Part model, mm, in its own coordinate system. A direction names the side the tool comes from. Coordinates: 2 decimals unless noted, no trailing zeros. Loops run counter-clockwise (first coordinate to the right, second up) from the corner with the lowest first, then second, coordinate; pieces in that order, holes last. Notation, with made-up numbers: (77.5, 22) - (98.5, 22) arc R32 ccw to (98.5, 48) - close; hole circle Ø9 at (81.5, -14.5). An arc over 180 degrees is marked (long way). Use a Markdown table: item, result. Add a question column.
1) Probe probe 1 along Z at (x, y) = (3, -5.5); probe 2 along Z at (x, y) = (-9, 2.75); probe 3 along Y at (x, z) = (-7, 4.5). List the from-to ranges inside material, lowest first. Write a range as [from, to].
2) Band-saw the part on B-B (z = -0.5). Give the cut face in (x, y).
3) Band-saw the part on C-C (x = -8). Give the cut face in (y, z).
4) Band-saw the part on A-A (z = -6.5). Give the cut face in (x, y), plus the area to 3 significant figures.
5) Drop flat-ended pins along their axis: P1, Ø1.1, axis at y = -2.5, z = 7.5, coming from the -X side; P2, Ø1, axis at x = -2, z = -0.5, coming from the -Y side; P3, Ø2.5, axis at x = -8, z = 5.5, coming from the +Y side. Give the stop position or say it passes through.
6) Pull direction X, two halves, no side cores. Call faces 1 (the face through (-11.75, -4, 0)), 2 (the face through (7, -4, 4)), 3 (the face through (-4, 1, -3)): +X half, -X half, draft (parallel to the pull), parting line (faces both ways), or undercut.
7) Tool access for faces 4 (the face through (-3.94, 1.79, -5.46)), 5 (the face through (6.036, -4.5, 7.5)), 6 (the face through (0.75, 4, -6)), 7 (the face through (1.65, 7.39, -5.46)): list every direction of +Z, -Z, +X, -X, +Y, -Y with a clear straight run to the whole face (end or side of a thin tool).
Autodesk Inventor part; units mm, degrees
ref_plane "YZ Plane" through (0, 0, 0) normal (1, 0, 0) x (0, 1, 0)
ref_plane "XZ Plane" through (0, 0, 0) normal (0, 1, 0) x (-1, 0, 0)
ref_plane "XY Plane" through (0, 0, 0) normal (0, 0, 1) x (1, 0, 0)
sketch "스케치1" plane through (0, 0, 0) normal (0, 0, 1) x (1, 0, 0)
  line L0 (-11.75, 8.25) -> (11.75, 8.25)
  line L1 (11.75, 8.25) -> (11.75, -8.25)
  line L2 (11.75, -8.25) -> (-11.75, -8.25)
  line L3 (-11.75, -8.25) -> (-11.75, 8.25)
  line L4 (-11.75, 8.25) -> (11.75, -8.25) construction
  line L5 (11.75, 8.25) -> (-11.75, -8.25) construction
  line L6 (-11.75, -4.25) -> (0.75, -4.25)
  line L7 (0.75, -4.25) -> (0.75, 8.25)
  circle A0 centre (-6.25, 2.75) radius 2.5
  point P0 (0, 0)
  dimension "d0" = 23.5
  dimension "d1" = 16.5
  dimension "d3" = 4
  dimension "d4" = 12.5
  dimension "d5" = 5
  dimension "d6" = 11
  dimension "d7" = 18
extrude "돌출1" add sketch "스케치1" along normal mid plane 16 contours L0 L1 L2 L3 L6 L7 | A0
extrude "돌출2" add sketch "스케치1" along normal mid plane 6 contours L0 L7 L6 L3
ref_plane "작업 평면1" through (0, 0, 0) normal (0, 0, 1) x (1, 0, 0)
sketch "스케치2" plane through (0, 0, 0) normal (0, 0, 1) x (1, 0, 0)
  line L0 (11.75, 8.25) -> (11.75, -8.25)
  line L1 (11.75, 5.75) -> (-3.25, -8.25)
  line L2 (-11.75, -8.25) -> (-11.75, -4.25)
  line L3 (11.75, -8.25) -> (-11.75, -8.25)
  point P0 (0, 0)
  dimension "d12" = 2.5
  dimension "d13" = 8.5
  dimension "d14" = 0
extrude "돌출3" cut sketch "스케치2" along normal mid plane 8
fillet "모깎기1" radius 3 2 edges at (0.75, 8.25, 5.5) (0.75, 8.25, -5.5)
fillet "모깎기2" radius 5.5 1 edges at (-11.75, 8.25, 0)
fillet "모깎기3" radius 7 2 edges at (0.75, -4.25, 5.5) (0.75, -4.25, -5.5)
sketch "스케치3" plane through (0, 0, 8) normal (0, 0, 1) x (1, 0, 0)
  line L0 (0.5954, -0.2053) -> (15.6035, -0.2053) construction
  line L1 (15.6035, -0.2053) -> (15.6035, -10.6024) construction
  line L2 (15.6035, -10.6024) -> (0.5954, -10.6024) construction
  line L3 (0.5954, -10.6024) -> (0.5954, -0.2053) construction
  spline S0 degree 2 poles (0.9131, -2.6219) (0.9131, -2.083) (1.2648, -1.1867) (1.5711, -0.8633) knots 0 0 0 1 2 2 2
  spline S1 degree 2 poles (1.5711, -0.8633) (1.8604, -0.5513) (2.7056, -0.2053) (3.1368, -0.2053) knots 0 0 0 1 2 2 2
  spline S2 degree 2 poles (3.1368, -0.2053) (3.6189, -0.2053) (4.4017, -0.5287) (4.691, -0.835) knots 0 0 0 1 2 2 2
  spline S3 degree 2 poles (4.691, -0.835) (5.0541, -1.2207) (5.4512, -2.4687) (5.4512, -3.4274) knots 0 0 0 1 2 2 2
  spline S4 degree 2 poles (5.4512, -3.4274) (5.4512, -4.2953) (5.0598, -5.8496) (4.6797, -6.3658) knots 0 0 0 1 2 2 2
  spline S5 degree 2 poles (4.6797, -6.3658) (4.2769, -6.9103) (3.1424, -7.4833) (2.3142, -7.4833) knots 0 0 0 1 2 2 2
  spline S6 degree 2 poles (2.3142, -7.4833) (2.127, -7.4833) (1.7016, -7.4436) (1.5201, -7.3868) knots 0 0 0 1 2 2 2
  line L4 (1.5201, -7.3868) -> (1.5201, -6.4849)
  line L5 (1.5201, -6.4849) -> (1.5654, -6.4849)
  spline S7 degree 2 poles (1.5654, -6.4849) (1.6846, -6.553) (2.1838, -6.6721) (2.439, -6.6721) knots 0 0 0 1 2 2 2
  spline S8 degree 2 poles (2.439, -6.6721) (3.358, -6.6721) (4.4074, -5.4582) (4.4812, -4.335) knots 0 0 0 1 2 2 2
  spline S9 degree 2 poles (4.4812, -4.335) (4.1068, -4.5902) (3.4261, -4.8228) (3.0233, -4.8228) knots 0 0 0 1 2 2 2
  spline S10 degree 2 poles (3.0233, -4.8228) (2.6376, -4.8228) (1.9966, -4.6526) (1.6732, -4.4087) knots 0 0 0 1 2 2 2
  spline S11 degree 2 poles (1.6732, -4.4087) (1.2988, -4.1194) (0.9131, -3.2402) (0.9131, -2.6219) knots 0 0 0 1 2 2 2
  spline S12 degree 2 poles (4.5039, -3.2175) (4.5039, -2.5084) (4.2429, -1.6121) (4.0103, -1.3682) knots 0 0 0 1 2 2 2
  spline S13 degree 2 poles (4.0103, -1.3682) (3.8061, -1.1413) (3.3807, -0.9711) (3.1311, -0.9711) knots 0 0 0 1 2 2 2
  spline S14 degree 2 poles (3.1311, -0.9711) (2.5525, -0.9711) (1.8661, -1.7993) (1.8661, -2.5821) knots 0 0 0 1 2 2 2
  spline S15 degree 2 poles (1.8661, -2.5821) (1.8661, -3.0246) (2.093, -3.5975) (2.3426, -3.8018) knots 0 0 0 1 2 2 2
  spline S16 degree 2 poles (2.3426, -3.8018) (2.5241, -3.9492) (2.9722, -4.0457) (3.2332, -4.0457) knots 0 0 0 1 2 2 2
  spline S17 degree 2 poles (3.2332, -4.0457) (3.5338, -4.0457) (4.2259, -3.8358) (4.4868, -3.6599) knots 0 0 0 1 2 2 2
  spline S18 degree 2 poles (4.4868, -3.6599) (4.4925, -3.5919) (4.5039, -3.3593) (4.5039, -3.2175) knots 0 0 0 1 2 2 2
  line L6 (10.8628, -4.9419) -> (10.029, -4.9419)
  line L7 (10.029, -4.9419) -> (10.029, -7.3471)
  line L8 (10.029, -7.3471) -> (9.127, -7.3471)
  line L9 (9.127, -7.3471) -> (9.127, -4.9419)
  line L10 (9.127, -4.9419) -> (6.0355, -4.9419)
  line L11 (6.0355, -4.9419) -> (6.0355, -3.9549)
  line L12 (6.0355, -3.9549) -> (9.1667, -0.3471)
  line L13 (9.1667, -0.3471) -> (10.029, -0.3471)
  line L14 (10.029, -0.3471) -> (10.029, -4.1875)
  line L15 (10.029, -4.1875) -> (10.8628, -4.1875)
  line L16 (10.8628, -4.1875) -> (10.8628, -4.9419)
  line L17 (9.127, -4.1875) -> (9.127, -1.4533)
  line L18 (9.127, -1.4533) -> (6.7729, -4.1875)
  line L19 (6.7729, -4.1875) -> (9.127, -4.1875)
  point P0 (0, 0)
extrude "돌출4" cut sketch "스케치3" against normal blind 1
properties part number "1번부품"
Answer block:
| question | item | result |
|---|---|---|
| 1 | probe 1 | [-8, -4], [4, 8] |
| 1 | probe 2 | [-3, 3] |
| 1 | probe 3 | [-8.25, -4.25], [0.37, 5.13] |
| 2 | outline | (-11.75, -8.25) - (-3.25, -8.25) - (11.75, 5.75) - (11.75, 8.25) - (-6.25, 8.25) arc R5.5 ccw to (-11.75, 2.75) - close |
| 3 | outline | (-8.25, -8) - (-4.25, -8) - (-4.25, -3) - (0.96, -3) - (0.96, -8) - (4.54, -8) - (4.54, -3) - (7.96, -3) - (7.96, 3) - (4.54, 3) - (4.54, 8) - (0.96, 8) - (0.96, 3) - (-4.25, 3) - (-4.25, 8) - (-8.25, 8) - close |
| 4 | outline | (-11.75, -8.25) - (11.75, -8.25) - (11.75, 8.25) - (3.75, 8.25) arc R3 ccw to (0.75, 5.25) - (0.75, 2.75) arc R7 cw to (-6.25, -4.25) - (-11.75, -4.25) - close; circle Ø5 at (-6.25, 2.75) |
| 4 | area | 260 mm2 |
| 5 | P1 | x = -2.33 |
| 5 | P2 | y = -7.55 |
| 5 | P3 | y = 5.2 |
| 6 | face 1 | -X half |
| 6 | face 2 | draft |
| 6 | face 3 | undercut |
| 7 | face 4 | -Z |
| 7 | face 5 | +Z |
| 7 | face 6 | -Z, +Y |
| 7 | face 7 | -Z, -X, +Y |
